Here's how the part is built. I have some questions about the finished solid (model axes, mm). Face numbers are marked on the shaded views. Coordinates: 2 decimals unless noted, no trailing zeros. Loops run counter-clockwise (first coordinate to the right, second up) from the corner with the lowest first, then second, coordinate; pieces in that order, holes last.
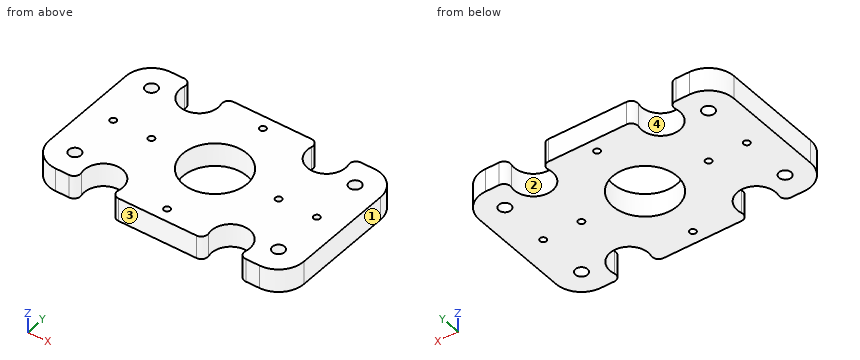
```python
from build123d import *

# Parameters (mm, degrees)
SKETCH1_W                       = 38.1
SKETCH1_H                       = 38.1
BOSS_EXTRUDE1_DEPTH             = 5.8
SKETCH2_R                       = 8
CUT_EXTRUDE1_DEPTH              = 12.7
SKETCH4_R                       = 0.79375
CUT_EXTRUDE3_DEPTH              = 55.19280395
SKETCH6_W                       = 12.7
SKETCH6_H                       = 38.1
BOSS_EXTRUDE2_DEPTH             = 5.8
CUT_EXTRUDE2_DEPTH              = 64.764331722
M3X0_5_TAPPED_HOLE1_D           = 2.5
M3X0_5_TAPPED_HOLE1_DEPTH       = 7.5
M3X0_5_TAPPED_HOLE1_CBORE_D     = 3
M3X0_5_TAPPED_HOLE1_CBORE_DEPTH = 6
M3X0_5_TAPPED_HOLE1_TIP         = 0.751075774
SKETCH9_R                       = 0.79375
CUT_EXTRUDE4_DEPTH              = 64.764331722
FILLET1_R                       = 6.35
FILLET2_R                       = 1.5875


with BuildPart() as part:
    # Sketch1 → Boss-Extrude1 (new body)
    with BuildSketch(Plane.XY):
        with Locations((-19.05, 19.05)):
            Rectangle(SKETCH1_W, SKETCH1_H)
    extrude(amount=BOSS_EXTRUDE1_DEPTH)

    # Sketch2 → Cut-Extrude1 (cut)
    with BuildSketch(Plane.XY.offset(5.8)):
        with Locations((-19.05, 19.05)):
            Circle(SKETCH2_R)
    extrude(amount=-CUT_EXTRUDE1_DEPTH, mode=Mode.SUBTRACT)

    # Sketch4 → Cut-Extrude3 (cut, through all)
    with BuildSketch(Plane.XY.offset(5.8)):
        with Locations((-34.925, 19.05)):
            Circle(SKETCH4_R)
        with Locations((-19.05, 34.925)):
            Circle(SKETCH4_R)
        with Locations((-3.175, 19.05)):
            Circle(SKETCH4_R)
        with Locations((-19.05, 3.175)):
            Circle(SKETCH4_R)
    extrude(amount=-CUT_EXTRUDE3_DEPTH, mode=Mode.SUBTRACT)

    # Sketch6 → Boss-Extrude2 (add, through all)
    with BuildSketch(Plane.XY.offset(5.8)):
        with Locations((6.35, 19.05)):
            Rectangle(SKETCH6_W, SKETCH6_H)
        with Locations((-44.45, 19.05)):
            Rectangle(SKETCH6_W, SKETCH6_H)
    extrude(amount=-BOSS_EXTRUDE2_DEPTH)

    # Sketch3 → Cut-Extrude2 (cut, through all)
    with BuildSketch(Plane.XY.offset(5.8)):
        with BuildLine():
            Line((-38.1, 38.1), (-31.375242086, 38.1))
            ThreePointArc((-31.375242086, 38.1), (-34.925, 30.1625), (-38.474757914, 38.1))
            Line((-38.474757914, 38.1), (-38.1, 38.1))
        make_face()
        with BuildLine():
            Line((0, 38.1), (-6.724757914, 38.1))
            ThreePointArc((-6.724757914, 38.1), (-3.175, 30.1625), (0.374757914, 38.1))
            Line((0.374757914, 38.1), (0, 38.1))
        make_face()
        with BuildLine():
            Line((0, 0), (-6.724757914, 0))
            ThreePointArc((-6.724757914, 0), (-3.175, 7.9375), (0.374757914, 0))
            Line((0.374757914, 0), (0, 0))
        make_face()
        with BuildLine():
            Line((-38.1, 0), (-31.375242086, 0))
            ThreePointArc((-31.375242086, 0), (-34.925, 7.9375), (-38.474757914, 0))
            Line((-38.474757914, 0), (-38.1, 0))
        make_face()
    extrude(amount=-CUT_EXTRUDE2_DEPTH, mode=Mode.SUBTRACT)

    # M3x0.5 Tapped Hole1
    with Locations(Plane.XY.offset(5.8)):
        with Locations((-44.45, 31.75), (6.35, 31.75), (6.35, 6.35), (-44.45, 6.35)):
            CounterBoreHole(M3X0_5_TAPPED_HOLE1_D / 2, M3X0_5_TAPPED_HOLE1_CBORE_D / 2, M3X0_5_TAPPED_HOLE1_CBORE_DEPTH, depth=M3X0_5_TAPPED_HOLE1_DEPTH)
            with Locations((0, 0, -(M3X0_5_TAPPED_HOLE1_DEPTH + M3X0_5_TAPPED_HOLE1_TIP / 2))):  # 118° drill point
                Cone(0, M3X0_5_TAPPED_HOLE1_D / 2, M3X0_5_TAPPED_HOLE1_TIP, mode=Mode.SUBTRACT)

    # Sketch9 → Cut-Extrude4 (cut, through all)
    with BuildSketch(Plane.XY.offset(5.8)):
        with Locations((-44.45, 19.05)):
            Circle(SKETCH9_R)
        with Locations((6.35, 19.05)):
            Circle(SKETCH9_R)
    extrude(amount=-CUT_EXTRUDE4_DEPTH, mode=Mode.SUBTRACT)

    # Fillet1
    fillet1_edges = [part.edges().sort_by_distance(p)[0] for p in [
        (12.7, 38.1, 2.9),
        (12.7, 0, 2.9),
        (-50.8, 0, 2.9),
        (-50.8, 38.1, 2.9),
    ]]
    fillet(fillet1_edges, radius=FILLET1_R)

    # Fillet2
    fillet2_edges = [part.edges().sort_by_distance(p)[0] for p in [
        (-38.474757914, 38.1, 2.9),
        (-31.375242086, 38.1, 2.9),
        (0.374757914, 0, 2.9),
        (-6.724757914, 0, 2.9),
        (0.374757914, 38.1, 2.9),
        (-6.724757914, 38.1, 2.9),
        (-38.474757914, 0, 2.9),
        (-31.375242086, 0, 2.9),
    ]]
    fillet(fillet2_edges, radius=FILLET2_R)


solid = part.part
```
1. We'd pull the mould along Y, two halves only. Please class the marked faces 1, 2, 3 and 4: +Y half, -Y half, draft (parallel to the pull), parting line (faces both ways), or undercut.
2. I want a section at B-B (y = 19.05). Please give me the cut outline in (x, z).
3. I need wall thicknesses on line 1 along Y through (x, z) = (-44.45, 3.7); line 2 along Y through (x, z) = (-19.05, 1.85); line 3 along X through (y, z) = (4.5, 4.85). Which ranges of each line are inside material? Lowest first, please.
4. I want a section at A-A (x = -19.05). Please give me the cut outline in (y, z), then the cut area to 3 significant figures.
5. I want a section at C-C (z = 1.95). Give the number of separate pieces and of enclosed holes in the cut face, then the cut area to 3 significant figures.
6. For pin 1 (1 mm diameter, centred on x = -19.05, y = 3.175, fed in from -Z); pin 2 (3 mm diameter, centred on y = 4, z = 2.5, fed in from +X), each with a flat end and sliding along its axis, tell me the tip position at first contact or that it passes through.
7. I want a section at D-D (x = -32.5). Please give me the cut outline in (y, z).
Response values:
1. face 1: draft
1. face 2: undercut
1. face 3: -Y half
1. face 4: undercut
2. outline: (-50.8, 0) - (-45.24, 0) - (-45.24, 5.8) - (-50.8, 5.8) - close; (-43.66, 0) - (-35.72, 0) - (-35.72, 5.8) - (-43.66, 5.8) - close; (-34.13, 0) - (-27.05, 0) - (-27.05, 5.8) - (-34.13, 5.8) - close; (-11.05, 0) - (-3.97, 0) - (-3.97, 5.8) - (-11.05, 5.8) - close; (-2.38, 0) - (5.56, 0) - (5.56, 5.8) - (-2.38, 5.8) - close; (7.14, 0) - (12.7, 0) - (12.7, 5.8) - (7.14, 5.8) - close
3. line 1: y = 0 to 4.85, 7.85 to 18.26, 19.84 to 30.25, 33.25 to 38.1
3. line 2: y = 0 to 2.38, 3.97 to 11.05, 27.05 to 34.13, 35.72 to 38.1
3. line 3: x = -50.52 to -39.5, -30.35 to -7.75, 1.4 to 12.42
4. outline: (0, 0) - (2.38, 0) - (2.38, 5.8) - (0, 5.8) - close; (3.97, 0) - (11.05, 0) - (11.05, 5.8) - (3.97, 5.8) - close; (27.05, 0) - (34.13, 0) - (34.13, 5.8) - (27.05, 5.8) - close; (35.72, 0) - (38.1, 0) - (38.1, 5.8) - (35.72, 5.8) - close
4. area: 110 mm2
5. separate pieces: 1
5. enclosed holes: 11
5. area: 1,880 mm2
6. pin 1: passes through
6. pin 2: stops at x = 12.64
7. outline: (7.27, 0) - (30.83, 0) - (30.83, 5.8) - (7.27, 5.8) - close
